Design review of the part built by this model. Coordinates are the model's own, in mm. Face numbers are marked on the shaded views. A direction names the side the tool comes from. Give positions to 0.01 mm unless a question says otherwise; leave off trailing zeros. Order: outer loops, then holes, each group sorted by start corner. A loop starts at its lowest first (then second) coordinate and runs counter-clockwise, first axis right, second up.
```python
from build123d import *

# Parameters (mm, degrees)
F3_DEPTH  = 10
F4_DEPTH  = 100
F1_W      = 17.366
F1_H      = 36.154188
F5_DEPTH  = 100
F6_W      = 40
F6_H      = 60
F7_DEPTH  = 10
F8_W      = 40
F8_H      = 60
F9_DEPTH  = 10
F10_W     = 40
F10_H     = 60
F11_DEPTH = 10
F12_W     = 40
F12_H     = 60
F12_W_2   = 30
F12_H_2   = 50
F13_DEPTH = 10
F14_W     = 15
F14_H     = 40
F14_W_2   = 55
F14_H_2   = 60
F15_DEPTH = 10
F16_W     = 80
F16_H     = 70
F17_DEPTH = 10
F18_W     = 30
F18_H     = 70
F18_H_2   = 10
F19_DEPTH = 10
F20_W     = 30
F20_H     = 70
F20_H_2   = 10
F21_DEPTH = 10
F22_W     = 30
F22_H     = 70
F22_H_2   = 10
F23_DEPTH = 10
F24_W     = 30
F24_H     = 70
F25_DEPTH = 10
F26_R     = 5
F27_W     = 45
F27_H     = 70
F28_DEPTH = 5.6
F29_W     = 55
F29_H     = 70
F30_DEPTH = 8
F31_W     = 64.428788
F31_H     = 70
F32_DEPTH = 10
F33_W     = 30
F33_H     = 70
F34_DEPTH = 10


with BuildPart() as f3:
    # F2 (on Top) → F3 (new body)
    with BuildSketch(Plane.XY):
        Polygon((95.242359, 211.719842), (-138.729709, 211.719842), (-138.342458, 131.481439), (-108.129827, 131.481439), (-108.046199, 94.60168), (-87.173399, 94.649011), (-86.914142, -19.682718), (-137.61172, -19.927398), (-137.295023, -85.54685), (-137.905847, -85.549798), (-137.633327, -142.015695), (144.48047, -142.015695), (144.48047, 61.8671), (113.558467, 61.8671), (113.558467, 138.765142), (124.934341, 138.765142), (124.934341, 192.200884), (95.242359, 192.200884), align=None)
    extrude(amount=F3_DEPTH)

    # F0 (on Top) → F4 (join)
    with BuildSketch(Plane.XY):
        Polygon((97.288959, 214.708266), (-141.752276, 214.708266), (-141.752276, -145.291734), (148.247724, -145.291734), (148.247724, 64.708266), (118.247724, 64.708266), (118.247724, 132.413622), (128.247724, 132.413622), (128.247724, 190.051958), (128.247724, 193.735838), (97.288959, 193.735838), align=None)
        Polygon((0, -140.291734), (-136.752276, -140.291734), (-136.752276, -24.433134), (0, -24.433134), (0, -134.701237), align=None, mode=Mode.SUBTRACT)
        Polygon((-136.752276, 135.399103), (-136.752276, 209.708266), (-52.510735, 209.708266), (-46.752276, 209.708266), (93.502745, 209.708266), (93.502745, 190.051958), (123.247724, 190.051958), (123.247724, 139.708266), (113.247724, 139.541012), (113.247724, 89.373782), (113.247724, 69.708266), (113.247724, 59.708266), (143.247724, 59.708266), (143.247724, 39.708266), (143.247724, -140.291734), (3.247724, -140.291734), (3.247724, -20.291734), (-80.555938, -20.291734), (-86.73545, -20.291734), (-136.752276, -20.291734), (-136.752276, 94.766736), (-136.752276, 99.708266), (-136.752276, 129.708266), align=None, mode=Mode.SUBTRACT)
    extrude(amount=F4_DEPTH)

    # F1 (on Top) → F5 (join)
    with BuildSketch(Plane.XY):
        Polygon((-46.381772, 210.111141), (-53.180333, 210.111141), (-53.180333, 138.726264), (-138.247326, 138.726264), (-138.247326, 130.567983), (-54.540046, 130.567983), (-54.540046, 54.424096), (0, 54.424096), (0, -19.680222), (-61.00649, -19.680222), (-61.00649, 21.1049), (-88.213228, 21.1049), (-87.853, -19.680222), (-137.235827, -19.680222), (-137.206597, -27.083231), (-13.823553, -27.083231), (-13.823553, -77.065498), (-13.823553, -142.692134), (-5.52455, -142.692134), (-5.52455, -77.065498), (0, -77.065498), (0, -143.060565), (8.686575, -143.060565), (8.686575, 34.028415), (90.665676, 34.028415), (145.648941, 34.028415), (145.648941, 37.734261), (90.665676, 37.734261), (90.665676, 41.440107), (112.807184, 41.440107), (112.807184, 55.10395), (137.995422, 55.10395), (143.29809, 55.10395), (144.269308, 61.888803), (114.873245, 61.888803), (114.873245, 71.072504), (0, 71.072504), (0, 61.888803), (-46.381772, 61.888803), align=None)
        with Locations((-74.89929, -1.603128)):
            Rectangle(F1_W, F1_H, mode=Mode.SUBTRACT)
        Polygon((105.549461, 45.731954), (8.765615, 45.731954), (8.765615, 65.555473), (90.949163, 65.555473), (96.314847, 65.555473), (105.549461, 65.555473), (105.549461, 55.10395), align=None, mode=Mode.SUBTRACT)
        Polygon((103.623547, 89.477897), (113.413647, 89.477897), (113.805249, 139.211625), (103.623547, 139.211625), align=None)
        Polygon((58.818936, -96.983925), (58.818936, -141.743556), (64.279255, -141.743556), (64.279255, -102.133363), (144.678116, -102.133363), (144.678116, -96.983925), align=None)
        Polygon((97.186632, 212.130934), (93.550943, 212.130934), (93.550943, 190.134004), (124.809749, 190.134004), (124.809749, 193.531185), (97.186632, 193.531185), align=None)
    extrude(amount=F5_DEPTH)

    # F6 (on face) → F7 (cut)
    with BuildSketch(Plane.YZ.offset(148.247724)):
        with Locations((-75.291734, 65)):
            Rectangle(F6_W, F6_H)
        with Locations((4.708266, 65)):
            Rectangle(F6_W, F6_H)
    extrude(amount=-F7_DEPTH, mode=Mode.SUBTRACT)

    # F8 (on face) → F9 (cut)
    with BuildSketch(Plane.YZ.offset(128.247724)):
        with Locations((162.413622, 65)):
            Rectangle(F8_W, F8_H)
    extrude(amount=-F9_DEPTH, mode=Mode.SUBTRACT)

    # F10 (on face) → F11 (cut)
    with BuildSketch(Plane.XZ.offset(145.291734)):
        with Locations((33.812322, 65)):
            Rectangle(F10_W, F10_H)
        with Locations((-71.752276, 65)):
            Rectangle(F10_W, F10_H)
    extrude(amount=-F11_DEPTH, mode=Mode.SUBTRACT)

    # F12 (on face) → F13 (cut)
    with BuildSketch(Plane(origin=(-141.752276, 0, 0), x_dir=(0, -1, 0), z_dir=(-1, 0, 0))):
        with Locations((49.433134, 65)):
            Rectangle(F12_W, F12_H)
        with Locations((-14.708266, 48)):
            Rectangle(F12_W_2, F12_H_2)
    extrude(amount=-F13_DEPTH, mode=Mode.SUBTRACT)

    # F14 (on face) → F15 (cut)
    with BuildSketch(Plane(origin=(0, 214.708266, 0), x_dir=(-1, 0, 0), z_dir=(0, 1, 0))):
        with Locations((95.571365, 70)):
            Rectangle(F14_W, F14_H)
        with Locations((115.571365, 70)):
            Rectangle(F14_W, F14_H)
        with Locations((-25.747724, 65)):
            Rectangle(F14_W_2, F14_H_2)
    extrude(amount=-F15_DEPTH, mode=Mode.SUBTRACT)

    # F16 (on face) → F17 (cut)
    with BuildSketch(Plane(origin=(0, 71.072504, 0), x_dir=(-1, 0, 0), z_dir=(0, 1, 0))):
        with Locations((-60, 45)):
            Rectangle(F16_W, F16_H)
    extrude(amount=-F17_DEPTH, mode=Mode.SUBTRACT)

    # F18 (on face) → F19 (cut)
    with BuildSketch(Plane(origin=(0, 61.888803, 0), x_dir=(-1, 0, 0), z_dir=(0, 1, 0))):
        with Locations((30, 45)):
            Rectangle(F18_W, F18_H)
        with Locations((30, 90)):
            Rectangle(F18_W, F18_H_2)
    extrude(amount=-F19_DEPTH, mode=Mode.SUBTRACT)

    # F20 (on face) → F21 (cut)
    with BuildSketch(Plane.XZ.offset(27.083231)):
        with Locations((-36.323553, 45)):
            Rectangle(F20_W, F20_H)
        with Locations((-36.323553, 90)):
            Rectangle(F20_W, F20_H_2)
    extrude(amount=-F21_DEPTH, mode=Mode.SUBTRACT)

    # F22 (on face) → F23 (cut)
    with BuildSketch(Plane.YZ.offset(8.686575)):
        with Locations((11.528415, 45)):
            Rectangle(F22_W, F22_H)
        with Locations((11.528415, 90)):
            Rectangle(F22_W, F22_H_2)
    extrude(amount=-F23_DEPTH, mode=Mode.SUBTRACT)

    # F24 (on face) → F25 (cut)
    with BuildSketch(Plane.XZ.offset(-130.567983)):
        with Locations((-69.528099, 45)):
            Rectangle(F24_W, F24_H)
    extrude(amount=-F25_DEPTH, mode=Mode.SUBTRACT)

    # F26
    f26_edges = [f3.edges().sort_by_distance(p)[0] for p in [
        (-54.540046, 54.424096, 55),
    ]]
    fillet(f26_edges, radius=F26_R)

    # F27 (on face) → F28 (cut)
    with BuildSketch(Plane.XZ.offset(-34.028415)):
        with Locations((115.747724, 45)):
            Rectangle(F27_W, F27_H)
    extrude(amount=-F28_DEPTH, mode=Mode.SUBTRACT)

    # F29 (on face) → F30 (cut)
    with BuildSketch(Plane(origin=(-13.823553, 0, 0), x_dir=(0, -1, 0), z_dir=(-1, 0, 0))):
        with Locations((107.791734, 45)):
            Rectangle(F29_W, F29_H)
    extrude(amount=-F30_DEPTH, mode=Mode.SUBTRACT)

    # F31 (on face) → F32 (cut)
    with BuildSketch(Plane(origin=(0, -96.983925, 0), x_dir=(-1, 0, 0), z_dir=(0, 1, 0))):
        with Locations((-101.03333, 45)):
            Rectangle(F31_W, F31_H)
    extrude(amount=-F32_DEPTH, mode=Mode.SUBTRACT)

    # F33 (on face) → F34 (cut)
    with BuildSketch(Plane.YZ.offset(-61.00649)):
        with Locations((-1.3951, 45)):
            Rectangle(F33_W, F33_H)
    extrude(amount=-F34_DEPTH, mode=Mode.SUBTRACT)


solid = f3.part
```
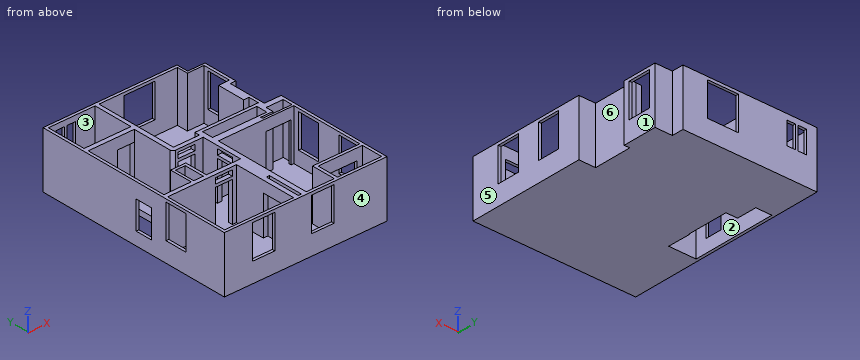
1. Take a section at D-D (y = -37.5). State the section outline as (x, z) points, then the cut area to 3 significant figures.
Recorded:
outline: (-141.75, 0) - (148.25, 0) - (148.25, 100) - (143.25, 100) - (143.25, 10) - (8.69, 10) - (8.69, 100) - (-13.82, 100) - (-13.82, 10) - (-136.75, 10) - (-136.75, 35) - (-141.75, 35) - close; (-141.75, 95) - (-136.75, 95) - (-136.75, 100) - (-141.75, 100) - close
area: 5,530 mm2
2. Draft analysis for pull direction Y (two halves, no side actions). For the marked faces 4, 5 and 6, state which applies: pulls with the +Y half, pulls with the -Y half, needs draft (parallel to the pull), parting line crosses it, or undercut.
Recorded:
face 4: pulls with the -Y half
face 5: needs draft
face 6: undercut
3. Take a section at B-B (y = -86). State the section outline as (x, z) points, then the cut area to 3 significant figures.
Recorded:
outline: (-141.75, 0) - (148.25, 0) - (148.25, 35) - (143.25, 35) - (143.25, 10) - (8.69, 10) - (8.69, 100) - (0, 100) - (0, 10) - (-5.52, 10) - (-5.52, 100) - (-13.82, 100) - (-13.82, 80) - (-5.82, 80) - (-5.82, 10) - (-136.75, 10) - (-136.75, 100) - (-141.75, 100) - close; (143.25, 95) - (148.25, 95) - (148.25, 100) - (143.25, 100) - close
area: 4,470 mm2
4. Take a section at C-C (x = 35.5). State the section outline as (y, z) points.
Recorded:
outline: (-145.29, 0) - (214.71, 0) - (214.71, 35) - (209.71, 35) - (209.71, 10) - (45.73, 10) - (45.73, 100) - (34.03, 100) - (34.03, 10) - (-140.29, 10) - (-140.29, 35) - (-145.29, 35) - close; (-145.29, 95) - (-140.29, 95) - (-140.29, 100) - (-145.29, 100) - close; (65.56, 80) - (71.07, 80) - (71.07, 100) - (65.56, 100) - close; (209.71, 95) - (214.71, 95) - (214.71, 100) - (209.71, 100) - close
5. Take a section at A-A (x = 76.5). State the section outline as (y, z) points, then the cut area to 3 significant figures.
Recorded:
outline: (-145.29, 0) - (214.71, 0) - (214.71, 100) - (209.71, 100) - (209.71, 10) - (45.73, 10) - (45.73, 100) - (34.03, 100) - (34.03, 10) - (-140.29, 10) - (-140.29, 100) - (-145.29, 100) - close; (-102.13, 80) - (-96.98, 80) - (-96.98, 100) - (-102.13, 100) - close; (65.56, 80) - (71.07, 80) - (71.07, 100) - (65.56, 100) - close
area: 5,770 mm2
6. For pin 1 (8.5 mm diameter, centred on x = -75, z = 63, fed in from -Y); pin 2 (4 mm diameter, centred on y = 213, z = 79, fed in from +X); pin 3 (5.5 mm diameter, centred on x = 145.5, y = -72.5, fed in from -Z); pin 4 (2 mm diameter, centred on y = 140, z = 16.5, fed in from +X), all flat-tipped, find the tip position at first contact; note any pin that passes through.
Recorded:
pin 1: stops at y = -27.08
pin 2: stops at x = 97.29
pin 3: stops at z = 0
pin 4: stops at x = 128.25
7. For line 1 along X through (y, z) = (15, 19); line 2 along X through (y, z) = (-115, 63); line 3 along X through (y, z) = (60, 91), list the stretches that pass through material, from the lowest coordinate up.
Recorded:
line 1: x = -141.75 to -136.75, -88.16 to -83.58, -66.22 to -61.01, 143.25 to 148.25
line 2: x = -141.75 to -136.75, -5.82 to -5.52, 0 to 8.69, 58.82 to 64.28, 143.25 to 148.25
line 3: x = -141.75 to -136.75, -54.54 to -45, -15 to 8.77, 105.55 to 148.25
8. Machinability: for the marked faces 1, 2 and 3, which of the approach directions +Z, -Z, +X, -X, +Y, -Y give a long, thin tool a straight path to every point of the face, cutting with its end or side? Answer none if there is none.
Recorded:
face 1: +Z, -Z, +X, +Y
face 2: +Z, -Z
face 3: +Z
